Drawing for the job (mm, zero at the part's lowest x, y, z). A direction names the side the tool comes from. Round coordinates to 2 decimals unless told otherwise and drop trailing zeros. Write each loop counter-clockwise with the first axis right and the second up, starting at its lowest first coordinate (ties: lowest second). Pieces come first, ordered by that corner, then holes. Notation, with made-up numbers: M 40,70.25 L 61,70.25 A28 cw 61,101.25 Z; hole C -6,27.25 d3. An arc over 180 degrees is marked long. Use a Markdown table: item, result. Add a question column.
1) Slice it at A-A on x = 11.5. Write the cut outline in (y, z).
2) Drop flat-ended pins along their axis: P1, Ø1, axis at y = 14.5, z = 3, coming from the +X side; P2, Ø4, axis at x = 11.5, y = 11.5, coming from the +Z side; P3, Ø1, axis at x = 19.5, z = 3, coming from the -Y side. Give the stop position or say it passes through.
3) Slice it at B-B on y = 11.5. Write the cut outline in (x, z).
4) Two-plate mould, pull along X, no slides. Class the marked faces 1, 2, 3 and 4: released by +X, released by -X, zero draft, split by the parting line, or undercut.
5) Wall check: probe 1 along Y at (x, z) = (11.5, 0.95); probe 2 along Z at (x, y) = (17.75, 4); probe 3 along X at (y, z) = (13.75, 4.3). Give the ranges that are in metal, low to high.
6) Which spindle directions (+Z, -Z, +X, -X, +Y, -Y) get a long thin tool onto all of the face, cutting with end or side? Do the marked faces 5, 6, 7 and 8. Say none if no direction does.
7) Slice it at D-D on y = 15.75. Write the cut outline in (x, z) (1 decimal).
8) Slice it at C-C on z = 2.55. Write the cut outline in (x, y).
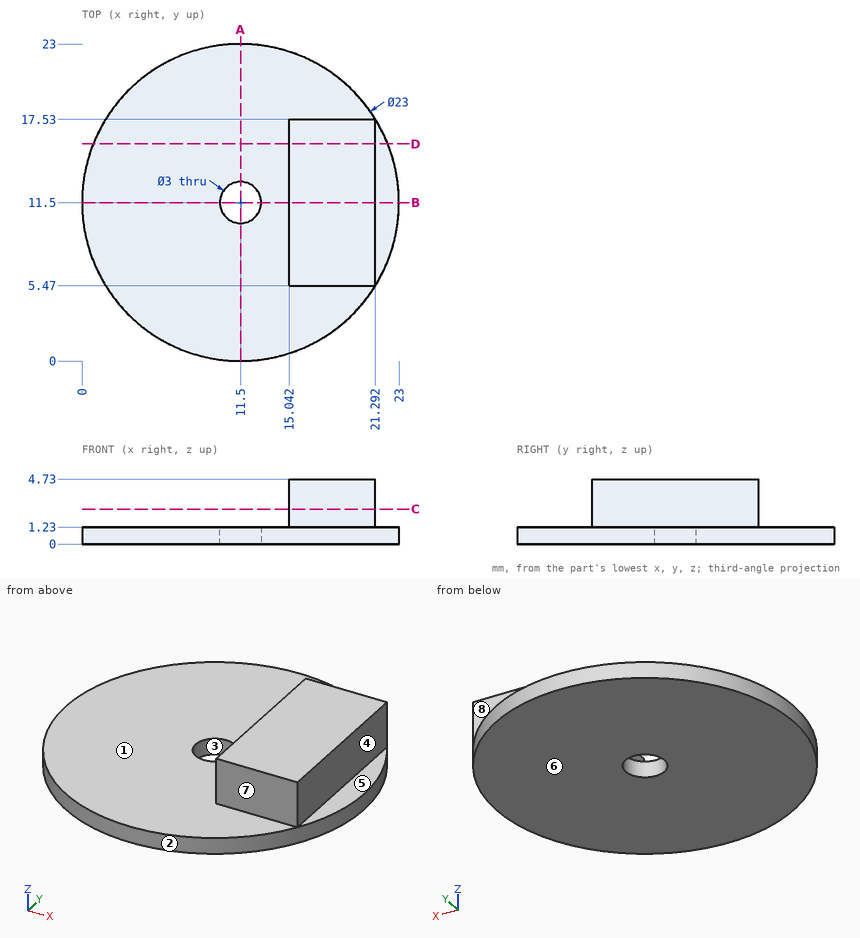
Entries:
| question | item | result |
|---|---|---|
| 1 | outline | M 0,0 L 10,0 L 10,1.23 L 0,1.23 Z; M 13,0 L 23,0 L 23,1.23 L 13,1.23 Z |
| 2 | P1 | stops at x = 21.29 |
| 2 | P2 | stops at z = 1.23 |
| 2 | P3 | stops at y = 5.47 |
| 3 | outline | M 0,0 L 10,0 L 10,1.23 L 0,1.23 Z; M 13,0 L 23,0 L 23,1.23 L 21.29,1.23 L 21.29,4.73 L 15.04,4.73 L 15.04,1.23 L 13,1.23 Z |
| 4 | face 1 | zero draft |
| 4 | face 2 | split by the parting line |
| 4 | face 3 | undercut |
| 4 | face 4 | released by +X |
| 5 | probe 1 | y = 0 to 10, 13 to 23 |
| 5 | probe 2 | z = 0 to 1.23 |
| 5 | probe 3 | x = 15.04 to 21.29 |
| 6 | face 5 | +Z, +X, +Y, -Y |
| 6 | face 6 | -Z, +X, -X, +Y, -Y |
| 6 | face 7 | +Z, +X, -X, -Y |
| 6 | face 8 | +Z, +X, -X, +Y |
| 7 | outline | M 0.8,0 L 22.2,0 L 22.2,1.2 L 21.3,1.2 L 21.3,4.7 L 15,4.7 L 15,1.2 L 0.8,1.2 Z |
| 8 | outline | M 15.04,5.47 L 21.29,5.47 L 21.29,17.53 L 15.04,17.53 Z |
